```python
from build123d import *

# Parameters (mm, degrees)
SKETCH3_R           = 1
BOSS_EXTRUDE1_DEPTH = 5
BOSS_EXTRUDE2_DEPTH = 7.5


with BuildPart() as part:
    # Sketch3 → Boss-Extrude1 (new body)
    with BuildSketch(Plane(origin=(0, 0, 0), x_dir=(1, 0, 0), z_dir=(0, 1, 0))):
        Circle(SKETCH3_R)
    extrude(amount=BOSS_EXTRUDE1_DEPTH)

    # Sketch4 → Boss-Extrude2 (add, symmetric)
    with BuildSketch(Plane(origin=(0, 0, 0), x_dir=(0, 0, -1), z_dir=(1, 0, 0))):
        with BuildLine():
            Line((-1, 0.158659908), (1, 0.158659908))
            ThreePointArc((1, 0.158659908), (1.158659908, 0), (1, -0.158659908))
            Line((1, -0.158659908), (-1, -0.158659908))
            ThreePointArc((-1, -0.158659908), (-1.158659908, 0), (-1, 0.158659908))
        make_face()
    extrude(amount=BOSS_EXTRUDE2_DEPTH, both=True)


solid = part.part
```
Verification items for the finished model (mm, model axes). A direction names the side the tool comes from. Coordinates: 2 decimals unless noted, no trailing zeros. Write each loop counter-clockwise with the first axis right and the second up, starting at its lowest first coordinate (ties: lowest second). Pieces come first, ordered by that corner, then holes. Notation, with made-up numbers: (30.5, 53) - (60.5, 53) arc R11 ccw to (60.5, 74) - close; hole circle Ø8 at (15.5, -17.75). An arc over 180 degrees is marked (long way). Write item = value, one per line.
Q1. Go/stop test with flat-tipped pins: pin 1 Ø1 at (y, z) = (4.5, 0) entering from -X; pin 2 Ø0.6 at (x, z) = (3.5, 0) entering from +Y. Record where each tip stops, or that it passes through.
Answer:
pin_1 = -1
pin_2 = 0.16
Q2. Material ranges on L1, parallel to Y at x = 3.75, z = -0.7; L2, parallel to X at y = 3.95, z = 0.1; L3, parallel to X at y = 3.95, z = -0.75, recorded low to high. Write a range as from..to.
Answer:
L1 = -0.16..0.16
L2 = -0.99..0.99
L3 = -0.66..0.66
Q3. Cross-section at B-B (y = 2.5). Enter the section's corners in (x, z).
Answer:
outline = circle Ø2 at (0, 0)
Q4. Cross-section at A-A (z = 0). Enter the section's corners in (x, y).
Answer:
outline = (-7.5, -0.16) - (7.5, -0.16) - (7.5, 0.16) - (1, 0.16) - (1, 5) - (-1, 5) - (-1, 0.16) - (-7.5, 0.16) - close
Q5. Cross-section at D-D (x = 0.75). Enter the section's corners in (y, z), plus the area to 3 significant figures.
Answer:
outline = (-0.16, -1) arc R0.16 ccw to (0.16, -1) - (0.16, -0.66) - (5, -0.66) - (5, 0.66) - (0.16, 0.66) - (0.16, 1) arc R0.16 ccw to (-0.16, 1) - close
area = 7.12 mm²
Q6. Access from +Z, -Z, +X, -X, +Y, -Y to the whole of each face (thin tool, end or side, straight path). Record for faces 1 (the face through (0, 3, 1)), 2 (the face through (0, -0.159, 0)).
Answer:
face_1 = +Y
face_2 = +Z, -Z, +X, -X, -Y
Q7. Cross-section at C-C (x = -4). Enter the section's corners in (y, z).
Answer:
outline = (-0.16, -1) arc R0.16 ccw to (0.16, -1) - (0.16, 1) arc R0.16 ccw to (-0.16, 1) - close
